For this review, take the finished solid that the model builds, in its own axes (mm). Face numbers are marked on the shaded views. Round coordinates to 2 decimals unless told otherwise and drop trailing zeros. Loops run counter-clockwise (first coordinate to the right, second up) from the corner with the lowest first, then second, coordinate; pieces in that order, holes last. Notation, with made-up numbers: (-38, 74.25) -> (3, 74.25) arc R29 ccw to (3, 103.25) -> close; hole circle Ø1 at (3, -38). An arc over 180 degrees is marked (long way). Use one line per item in the form item = value. Start each with the question number.
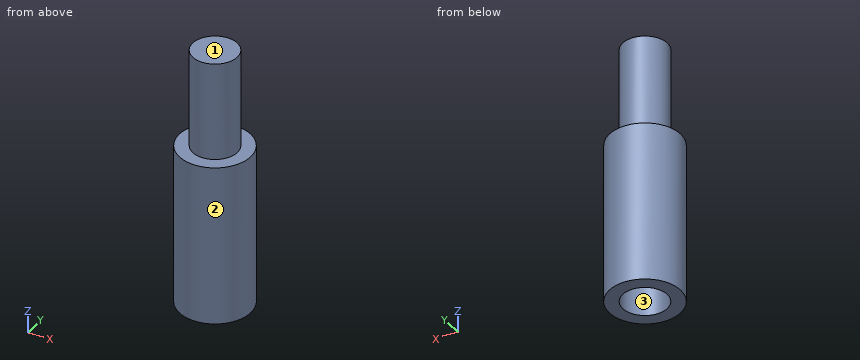
Autodesk Inventor part; units mm, degrees
ref_plane "YZ Plane" through (0, 0, 0) normal (1, 0, 0) x (0, 1, 0)
ref_plane "XZ Plane" through (0, 0, 0) normal (0, 1, 0) x (-1, 0, 0)
ref_plane "XY Plane" through (0, 0, 0) normal (0, 0, 1) x (1, 0, 0)
sketch "Sketch1" plane through (0, 0, 0) normal (0, 0, 1) x (1, 0, 0)
  circle A0 centre (0, 0) radius 1.25
  dimension "d0" = 2.5
extrude "Extrusion1" add sketch "Sketch1" along normal blind 14.5
sketch "Sketch3" plane through (0, 0, 0) normal (0, 0, -1) x (-1, 0, 0)
  circle A0 centre (0, 0) radius 2
  dimension "d6" = 4
extrude "Extrusion3" add sketch "Sketch3" against normal blind 9
sketch "Sketch4" plane through (0, 0, 0) normal (0, 0, -1) x (-1, 0, 0)
  circle A0 centre (0, 0) radius 1.25
  circle A1 centre (0, 0) radius 1.25
extrude "Extrusion4" cut sketch "Sketch4" against normal blind 5
properties part number "cannula_with_hole_v01"
Item 1: Take a section at C-C on z = 4.75. Give the boundary of the cut face in (x, y), plus the area to 3 significant figures.
Item 2: Take a section at A-A on y = 0. Give the boundary of the cut face in (x, z), plus the area to 4 significant figures.
Item 3: Draft analysis for pull direction Y (two halves, no side actions). For the marked faces 1, 2 and 3, state which applies: +Y half, -Y half, draft (parallel to the pull), parting line (faces both ways), or undercut.
Item 4: Wall thickness on line 1 (Y direction, x = 0, z = 3.4); line 2 (Z direction, x = 0.1, y = 0.45); line 3 (Z direction, x = 1.7, y = 0.1): over which ranges is each line inside the solid? List them lowest first.
Item 5: Take a section at D-D on z = 11.25. Give the boundary of the cut face in (x, y).
Item 6: For P1, Ø1, axis at x = 1.5, z = 4, coming from the -Y side; P2, Ø1.2, axis at x = 0, y = 0, coming from the -Z side, all flat-tipped, find the tip position at first contact; note any pin that passes through.
Results:
q1.outline = circle Ø4 at (0, 0); hole circle Ø2.5 at (0, 0)
q1.area = 7.66 mm2
q2.outline = (-2, 0) -> (-1.25, 0) -> (-1.25, 5) -> (1.25, 5) -> (1.25, 0) -> (2, 0) -> (2, 9) -> (1.25, 9) -> (1.25, 14.5) -> (-1.25, 14.5) -> (-1.25, 9) -> (-2, 9) -> close
q2.area = 37.25 mm2
q3.face_1 = draft
q3.face_2 = parting line
q3.face_3 = undercut
q4.line_1 = -2 to -1.25, 1.25 to 2
q4.line_2 = 5 to 14.5
q4.line_3 = 0 to 9
q5.outline = circle Ø2.5 at (0, 0)
q6.P1 = -1.73
q6.P2 = 5
